Solid Edge part; units mm, degrees
sketch "Sketch1" plane through (0, 0, 0) normal (0, -1, 0) x (1, 0, 0)
  line L0 (-10, 6) -> (10, 6)
  line L1 (10, 6) -> (10, -6)
  line L2 (10, -6) -> (-10, -6)
  line L3 (-10, -6) -> (-10, 6)
  dimension "D1" = 10
  dimension "D2" = 10
extrude "Protrusion1" add sketch "Sketch1" along normal blind 10
sketch "Sketch2" plane through (0, -10, 0) normal (0, -1, 0) x (1, 0, 0)
  line L0 (-10.5, 6.5) -> (10.5, 6.5)
  line L1 (10.5, 6.5) -> (10.5, -6.5)
  line L2 (10.5, -6.5) -> (-10.5, -6.5)
  line L3 (-10.5, -6.5) -> (-10.5, 6.5)
extrude "Wall" add sketch "Sketch2" along normal blind 1
sketch "Sketch3" plane through (0, -10.5, 4.5) normal (0, 0, 1) x (1, 0, 0)
  line L0 (8.5, -0.5) -> (-8.5, -0.5)
  arc A0 (5.5, -4.5) -> (-8.5, -0.5) centre (-8.5, -27) ccw
  line L1 (8.5, -0.5) -> (5.5, -4.5)
  dimension "D1" = 8.5
extrude "Button_Profile_Plane1" add sketch "Sketch3" against normal blind 9
sketch "Sketch4" plane through (0, 0, 0) normal (0, 1, 0) x (-1, 0, 0)
  line L0 (-4.75, -2.5) -> (-4.25, -2.5)
  line L1 (-4.25, -2.5) -> (-4.25, 2.5)
  line L2 (-4.25, 2.5) -> (-4.75, 2.5)
  line L3 (-4.75, 2.5) -> (-4.75, -2.5)
  line L4 (-0.25, -2.5) -> (0.25, -2.5)
  line L5 (0.25, -2.5) -> (0.25, 2.5)
  line L6 (0.25, 2.5) -> (-0.25, 2.5)
  line L7 (-0.25, 2.5) -> (-0.25, -2.5)
  dimension "D1" = 4.75
  dimension "D2" = 4.25
extrude "Electrics" add sketch "Sketch4" along normal blind 4
hole "Wire" at (-0.25, 2.8, 0) direction (1, 0, 0) diameter 1 end through all
properties material "ABS Plastic, high impact"
CAD build for the part. Positions are in the model's coordinates, mm. A direction names the side the tool comes from. Coordinates: 2 decimals unless noted, no trailing zeros. Loops run counter-clockwise (first coordinate to the right, second up) from the corner with the lowest first, then second, coordinate; pieces in that order, holes last. Notation, with made-up numbers: (57.5, 30.5) -> (108.5, 30.5) arc R28 ccw to (108.5, 59.5) -> close; hole circle Ø3 at (75.5, -12). An arc over 180 degrees is marked (long way). One line per item, written item: value.
1. Flat gauge pins, fed straight in: P1, Ø5, axis at y = -6, z = -1, coming from the +X side; P2, Ø2, axis at x = -2.5, y = -6, coming from the +Z side; P3, Ø4, axis at x = -5.5, y = -1, coming from the -Z side. Where does each tip first touch, or does it go through?
Answers:
P1: stops at x = 10
P2: stops at z = 6
P3: stops at z = -6
2. Which spindle directions (+Z, -Z, +X, -X, +Y, -Y) get a long thin tool onto all of the face, cutting with end or side? Do faces 4 (the face through (-0.25, 2, 0)), 5 (the face through (0, -11, -6)), 6 (the face through (0, -5, -6)), 7 (the face through (4, -12, 4.5)). Say none if no direction does.
Answers:
face 4: +Z, -Z, -X, +Y
face 5: -Y
face 6: -Z, +X, -X, +Y
face 7: +Z, +X, -X, -Y
3. Slice it at A-A on y = 2.8. Write the cut outline in (x, z).
Answers:
outline: (-0.25, -2.5) -> (0.25, -2.5) -> (0.25, -0.5) -> (-0.25, -0.5) -> close; (-0.25, 0.5) -> (0.25, 0.5) -> (0.25, 2.5) -> (-0.25, 2.5) -> close; (4.25, -2.5) -> (4.75, -2.5) -> (4.75, -0.5) -> (4.25, -0.5) -> close; (4.25, 0.5) -> (4.75, 0.5) -> (4.75, 2.5) -> (4.25, 2.5) -> close
4. Pull direction Z, two halves, no side cores. Call faces 1 (the face through (0, -10, -6.3)), 2 (the face through (4.496, 2.312, -0.108)), 3 (the face through (0, -5, 6)): pulls with the +Z half, pulls with the -Z half, needs draft (parallel to the pull), parting line crosses it, or undercut.
Answers:
face 1: needs draft
face 2: undercut
face 3: pulls with the +Z half
5. Slice it at D-D on x = -2. Write the cut outline in (y, z), and give its area (3 significant figures).
Answers:
outline: (-11.81, -4.5) -> (-11, -4.5) -> (-11, -6.5) -> (-10, -6.5) -> (-10, -6) -> (0, -6) -> (0, 6) -> (-10, 6) -> (-10, 6.5) -> (-11, 6.5) -> (-11, 4.5) -> (-11.81, 4.5) -> close
area: 140 mm^2
6. Drill centre lines: line 1 (X direction, y = 1.5, z = -2.25); line 2 (X direction, y = -1, z = 4); line 3 (Y direction, x = -0.05, z = 0). Where is each one in solid material? Low to high. Write a range as [from, to].
Answers:
line 1: x = [-0.25, 0.25], [4.25, 4.75]
line 2: x = [-10, 10]
line 3: y = [-12.38, 2.3], [3.3, 4]
7. Slice it at B-B on z = 0. Write the cut outline in (x, y), and give its area (3 significant figures).
Answers:
outline: (-10.5, -11) -> (-8.5, -11) arc R26.5 cw to (5.5, -15) -> (8.5, -11) -> (10.5, -11) -> (10.5, -10) -> (10, -10) -> (10, 0) -> (4.75, 0) -> (4.75, 2.3) -> (4.25, 2.3) -> (4.25, 0) -> (0.25, 0) -> (0.25, 2.3) -> (-0.25, 2.3) -> (-0.25, 0) -> (-10, 0) -> (-10, -10) -> (-10.5, -10) -> close; (-0.25, 3.3) -> (0.25, 3.3) -> (0.25, 4) -> (-0.25, 4) -> close; (4.25, 3.3) -> (4.75, 3.3) -> (4.75, 4) -> (4.25, 4) -> close
area: 248 mm^2
8. Slice it at C-C on z = -4.25. Write the cut outline in (x, y), and give its area (3 significant figures).
Answers:
outline: (-10.5, -11) -> (-8.5, -11) arc R26.5 cw to (5.5, -15) -> (8.5, -11) -> (10.5, -11) -> (10.5, -10) -> (10, -10) -> (10, 0) -> (-10, 0) -> (-10, -10) -> (-10.5, -10) -> close
area: 245 mm^2
